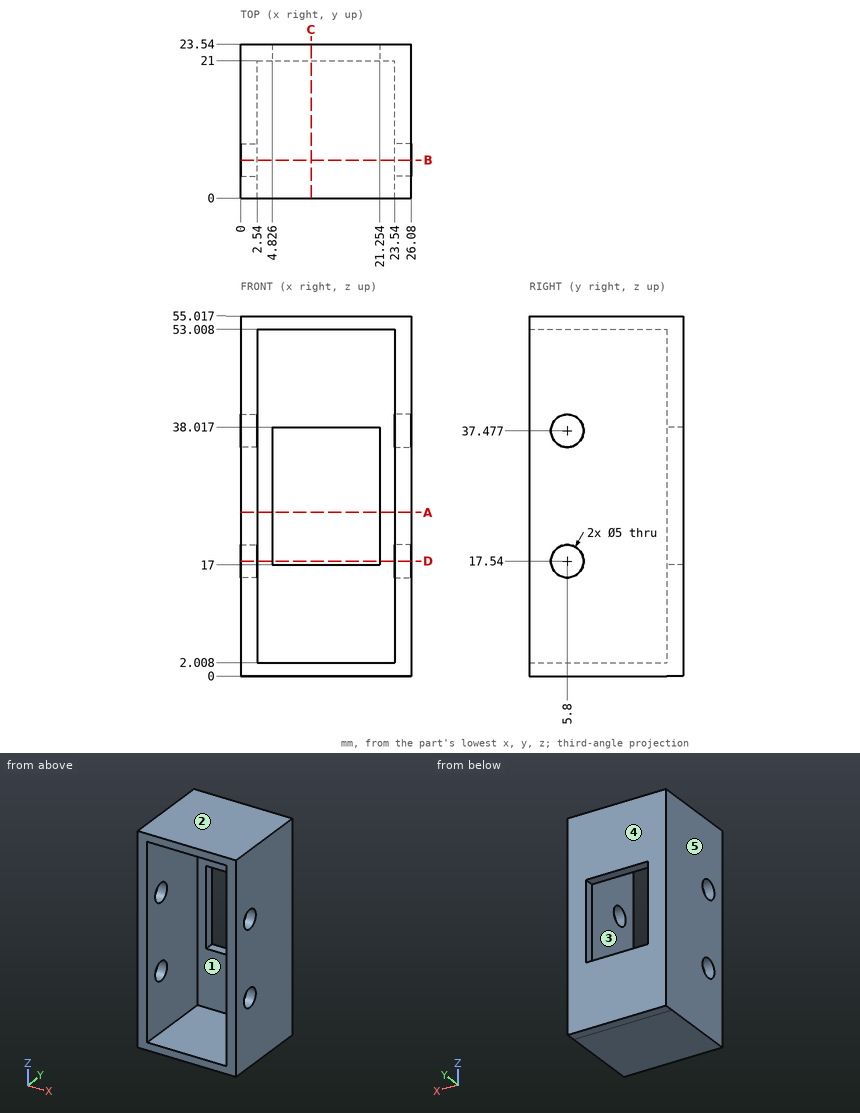
Here's the drawing with two shaded views (mm, measured from the low corner). I have some questions. A direction names the side the tool comes from. Coordinates: 2 decimals unless noted, no trailing zeros. Loops run counter-clockwise (first coordinate to the right, second up) from the corner with the lowest first, then second, coordinate; pieces in that order, holes last. Notation, with made-up numbers: (55, -29.75) -> (63, -29.75) arc R24 ccw to (63, 0.25) -> close; hole circle Ø7 at (-38, 25.5). An arc over 180 degrees is marked (long way). Put each result on its own line as item: value. Start each with the question number.
Q1. Thinking about a two-plate mould opening in X: for the marked faces 3, 4 and 5, which applies, pulls with the +X half, pulls with the -X half, needs draft (parallel to the pull), parting line crosses it, or undercut?
Q2. I'm going to push flat-ended pins straight in: P1, Ø4, axis at y = 5.8, z = 37.48, coming from the -X side; P2, Ø4, axis at x = 6, z = 44, coming from the -Y side. Where does each tip first touch, or does it pass through?
Q3. I want a section at D-D (z = 17.54). Write out the boundary of the cut face in (x, y), plus the area to 3 significant figures.
Q4. I want a section at C-C (x = 10.75). Write out the boundary of the cut face in (y, z), plus the area to 3 significant figures.
Q5. I want a section at A-A (z = 25). Write out the boundary of the cut face in (x, y), plus the area to 3 significant figures.
Q6. If I drill on line 1 (Z direction, x = 24.4, y = 5.8); line 2 (X direction, y = 7.5, z = 5); line 3 (Y direction, x = 24.75, z = 17.54), over which ranges is the centre line in solid material (lowest first)? Write a range as [from, to].
Q7. For the marked faces 1 and 2, which set-ups out of +Z, -Z, +X, -X, +Y, -Y let a thin tool reach every point of the face, with its end or its side?
Q8. I want a section at B-B (y = 5.8). Write out the boundary of the cut face in (x, z), plus the area to 3 significant figures.
Taken from the geometry:
1. face 3: undercut
1. face 4: needs draft
1. face 5: pulls with the -X half
2. P1: passes through
2. P2: stops at y = 21
3. outline: (0, 0) -> (2.54, 0) -> (2.54, 3.3) -> (0, 3.3) -> close; (0, 8.3) -> (2.54, 8.3) -> (2.54, 21) -> (4.83, 21) -> (4.83, 23.54) -> (0, 23.54) -> close; (21.25, 21) -> (23.54, 21) -> (23.54, 8.3) -> (26.08, 8.3) -> (26.08, 23.54) -> (21.25, 23.54) -> close; (23.54, 0) -> (26.08, 0) -> (26.08, 3.3) -> (23.54, 3.3) -> close
3. area: 106 mm2
4. outline: (0, 0) -> (23.54, 0) -> (23.54, 17) -> (21, 17) -> (21, 2.01) -> (0, 2.01) -> close; (0, 53.01) -> (21, 53.01) -> (21, 38.02) -> (23.54, 38.02) -> (23.54, 55.02) -> (0, 55.02) -> close
4. area: 171 mm2
5. outline: (0, 0) -> (2.54, 0) -> (2.54, 21) -> (4.83, 21) -> (4.83, 23.54) -> (0, 23.54) -> close; (21.25, 21) -> (23.54, 21) -> (23.54, 0) -> (26.08, 0) -> (26.08, 23.54) -> (21.25, 23.54) -> close
5. area: 131 mm2
6. line 1: z = [0, 15.04], [20.04, 34.98], [39.98, 55.02]
6. line 2: x = [0, 2.54], [23.54, 26.08]
6. line 3: y = [0, 3.3], [8.3, 23.54]
7. face 1: -Y
7. face 2: +Z, +X, -X, +Y, -Y
8. outline: (0, 0) -> (26.08, 0) -> (26.08, 15.04) -> (23.54, 15.04) -> (23.54, 2.01) -> (2.54, 2.01) -> (2.54, 15.04) -> (0, 15.04) -> close; (0, 20.04) -> (2.54, 20.04) -> (2.54, 34.98) -> (0, 34.98) -> close; (0, 39.98) -> (2.54, 39.98) -> (2.54, 53.01) -> (23.54, 53.01) -> (23.54, 39.98) -> (26.08, 39.98) -> (26.08, 55.02) -> (0, 55.02) -> close; (23.54, 20.04) -> (26.08, 20.04) -> (26.08, 34.98) -> (23.54, 34.98) -> close
8. area: 313 mm2
